Input: part model. Units: mm. Frame: model coordinates. Face numbers are marked on the shaded views. Give positions to 0.01 mm unless a question says otherwise; leave off trailing zeros. Loops run counter-clockwise (first coordinate to the right, second up) from the corner with the lowest first, then second, coordinate; pieces in that order, holes last. Notation, with made-up numbers: M 60,10.5 L 103,10.5 A18 cw 103,43.5 Z; hole C 6,70.5 d5. An arc over 180 degrees is marked long. Answer as a JSON object with one key per item and string values. Group by question number.
1) Section query C-C on y = 1.5. Return loops of the section in (x, z).
2) Draft query along Z for the marked faces 1, 2, 3 and 4. Return one class per face: +Z half, -Z half, draft (parallel to the pull), parting line (faces both ways), or undercut.
3) Ray query, L1, parallel to X at y = 4.25, z = 0; L2, parallel to X at y = 0.9, z = 0. Return the intervals inside material, ascending.
4) First-contact query: P1, Ø8.5, axis at x = 0, z = 0, coming from the -Y side; P2, Ø1, axis at x = 2, y = 6.5, coming from the -Z side; P3, Ø5, axis at x = 4, y = 8.5, coming from the +Z side; P4, Ø3, axis at x = -4, y = 7, coming from the +Z side. Flat tips, straight axial feed; report the tip coordinate or a pass-through.
5) Section query B-B on y = 2.5. Return loops of the section in (x, z).
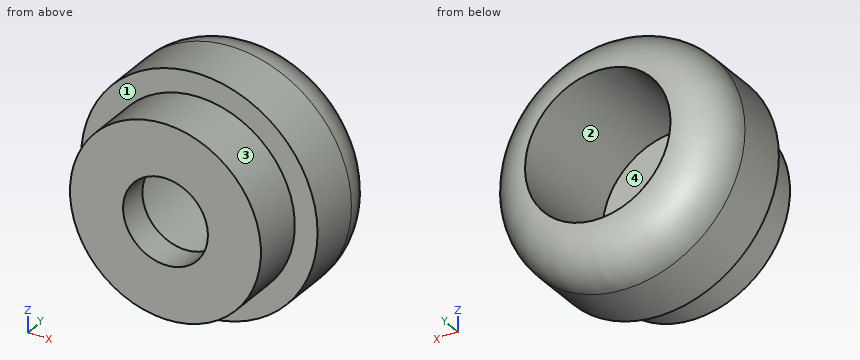
from build123d import *

# Parameters (mm, degrees)
SKETCH1_R               = 7.8
BOSS_EXTRUDE1_DEPTH     = 10
SKETCH2_R               = 4.8
CUT_EXTRUDE1_DEPTH      = 8
CUT_EXTRUDE2_DEPTH      = 1.5
CUT_EXTRUDE2_DEPTH_BACK = 14.626444878
SKETCH3_R               = 7.8
SKETCH3_R_2             = 6.3
SKETCH3_R_3             = 2.8
FILLET1_R               = 3


with BuildPart() as part:
    # Sketch1 → Boss-Extrude1 (new body)
    with BuildSketch(Plane(origin=(0, 0, 0), x_dir=(1, 0, 0), z_dir=(0, 1, 0))):
        with Locations(Location((0, 0, 0), (0, 0, 270))):
            Circle(SKETCH1_R)
    extrude(amount=BOSS_EXTRUDE1_DEPTH)

    # Sketch2 → Cut-Extrude1 (cut)
    with BuildSketch(Plane(origin=(0, 10, 0), x_dir=(1, 0, 0), z_dir=(0, 1, 0))):
        with Locations(Location((0, 0, 0), (0, 0, 270))):
            Circle(SKETCH2_R)
    extrude(amount=-CUT_EXTRUDE1_DEPTH, mode=Mode.SUBTRACT)

    # Sketch3 → Cut-Extrude2 (cut, two sides: drawn at the far end of the back side and taken through both)
    # profile 1 of 2: a face of its own
    with BuildSketch(Plane(origin=(0, 2, 0), x_dir=(1, 0, 0), z_dir=(0, 1, 0)).offset(-CUT_EXTRUDE2_DEPTH_BACK)):
        with Locations(Location((0, 0, 0), (0, 0, 270))):
            Circle(SKETCH3_R)
        with Locations(Location((0, 0, 0), (0, 0, 270))):
            Circle(SKETCH3_R_2, mode=Mode.SUBTRACT)
    # profile 2 of 2: a face of its own
    with BuildSketch(Plane(origin=(0, 2, 0), x_dir=(1, 0, 0), z_dir=(0, 1, 0)).offset(-CUT_EXTRUDE2_DEPTH_BACK)):
        with Locations(Location((0, 0, 0), (0, 0, 270))):
            Circle(SKETCH3_R_3)
    extrude(amount=CUT_EXTRUDE2_DEPTH + CUT_EXTRUDE2_DEPTH_BACK, mode=Mode.SUBTRACT)

    # Fillet1
    fillet1_edges = [part.edges().sort_by_distance(p)[0] for p in [
        (0, 10, -7.8),
    ]]
    fillet(fillet1_edges, radius=FILLET1_R - 0.0001)  # a hair under: the kernel refuses the full size


solid = part.part
Output:
{
 "1": {"outline": "C 0,0 d12.6; hole C 0,0 d5.6"},
 "2": {"face 1": "draft", "face 2": "undercut", "face 3": "parting line", "face 4": "undercut"},
 "3": {"L1": "x = -7.8 to -4.8, 4.8 to 7.8", "L2": "x = -6.3 to -2.8, 2.8 to 6.3"},
 "4": {"P1": "stops at y = 0", "P2": "stops at z = -7.65", "P3": "stops at z = 7.57", "P4": "stops at z = 7.39"},
 "5": {"outline": "C 0,0 d12.6; hole C 0,0 d9.6"}
}
